```python
from build123d import *

# Parameters (mm, degrees)
SKETCH1_R           = 50
BOSS_EXTRUDE1_DEPTH = 16
SKETCH2_R           = 50
SKETCH2_R_2         = 46.5
BOSS_EXTRUDE2_DEPTH = 1
SKETCH3_R           = 47
CUT_EXTRUDE1_DEPTH  = 10
SKETCH4_R           = 3.15
BOSS_EXTRUDE3_DEPTH = 7


with BuildPart() as part:
    # Sketch1 → Boss-Extrude1 (new body)
    with BuildSketch(Plane(origin=(0, 0, 0), x_dir=(1, 0, 0), z_dir=(0, 1, 0))):
        Circle(SKETCH1_R)
    extrude(amount=BOSS_EXTRUDE1_DEPTH)

    # Sketch2 → Boss-Extrude2 (add)
    with BuildSketch(Plane(origin=(0, 16, 0), x_dir=(1, 0, 0), z_dir=(0, 1, 0))):
        Circle(SKETCH2_R)
        Circle(SKETCH2_R_2, mode=Mode.SUBTRACT)
    extrude(amount=BOSS_EXTRUDE2_DEPTH)

    # Sketch3 → Cut-Extrude1 (cut)
    with BuildSketch(Plane.XZ):
        Circle(SKETCH3_R)
    extrude(amount=-CUT_EXTRUDE1_DEPTH, mode=Mode.SUBTRACT)

    # Sketch4 → Boss-Extrude3 (add)
    with BuildSketch(Plane(origin=(0, 0, 0), x_dir=(1, 0, 0), z_dir=(0, 1, 0))):
        with BuildLine():
            Line((-47.696960071, 15), (-70, 15))
            Line((-70, 15), (-70, -15))
            Line((-70, -15), (-47.696960071, -15))
            ThreePointArc((-47.696960071, -15), (-50, 0), (-47.696960071, 15))
        make_face()
        with Locations((-60, 0)):
            Circle(SKETCH4_R, mode=Mode.SUBTRACT)
        with BuildLine():
            Line((47.696960071, -15), (70, -15))
            Line((70, -15), (70, 15))
            Line((70, 15), (47.696960071, 15))
            ThreePointArc((47.696960071, 15), (50, 0), (47.696960071, -15))
        make_face()
        with Locations((60, 0)):
            Circle(SKETCH4_R, mode=Mode.SUBTRACT)
    extrude(amount=BOSS_EXTRUDE3_DEPTH)


solid = part.part
```
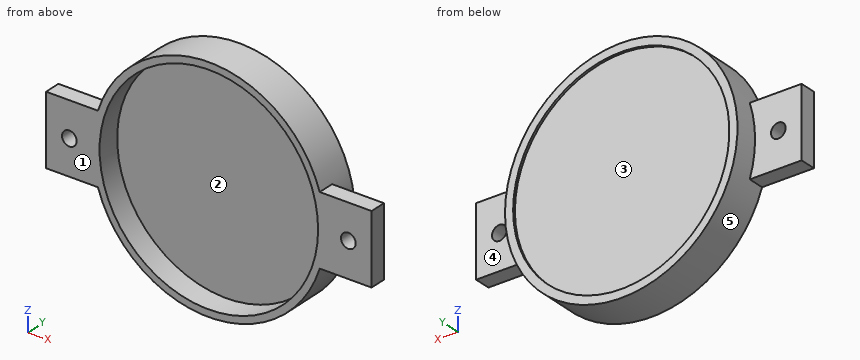
Verification items for the finished model (mm, model axes). Face numbers are marked on the shaded views. A direction names the side the tool comes from. Coordinates: 2 decimals unless noted, no trailing zeros. Loops run counter-clockwise (first coordinate to the right, second up) from the corner with the lowest first, then second, coordinate; pieces in that order, holes last. Notation, with made-up numbers: (-7.75, 48.25) -> (35.25, 48.25) arc R25 cw to (35.25, 82.25) -> close; hole circle Ø7 at (89.25, -4.75). An arc over 180 degrees is marked (long way). Put each result on its own line as item: value.
1. Section check A-A, the plane x = -60. Record the boundary of the cut face in (y, z).
Result set:
outline: (0, -15) -> (7, -15) -> (7, -3.15) -> (0, -3.15) -> close; (0, 3.15) -> (7, 3.15) -> (7, 15) -> (0, 15) -> close
2. Section check B-B, the plane z = 0. Record the boundary of the cut face in (x, y), then the cut area to 3 significant figures.
Result set:
outline: (-70, 0) -> (-63.15, 0) -> (-63.15, 7) -> (-70, 7) -> close; (-56.85, 0) -> (-47, 0) -> (-47, 10) -> (47, 10) -> (47, 0) -> (56.85, 0) -> (56.85, 7) -> (50, 7) -> (50, 17) -> (46.5, 17) -> (46.5, 16) -> (-46.5, 16) -> (-46.5, 17) -> (-50, 17) -> (-50, 7) -> (-56.85, 7) -> close; (63.15, 0) -> (70, 0) -> (70, 7) -> (63.15, 7) -> close
area: 859 mm^2
3. Mould release check, pull along Z, two halves, no side actions. Record for the marked faces 3, 4 and 5: pulls with the +Z half, pulls with the -Z half, needs draft (parallel to the pull), parting line crosses it, or undercut.
Result set:
face 3: undercut
face 4: needs draft
face 5: parting line crosses it
4. Tool access check on the marked faces 1 and 2. Record the directions out of +Z, -Z, +X, -X, +Y, -Y that give a thin tool (end or side, any length) a straight path to the whole face; none if there is none.
Result set:
face 1: +Z, -Z, +X, -X, -Y
face 2: -Y
5. Thickness scan on line 1 (Z direction, x = 0, y = 5.75); line 2 (Z direction, x = 0, y = 16.7); line 3 (Y direction, x = 43.5, z = 12). Record the ranges inside material, lowest first.
Result set:
line 1: z = -50 to -47, 47 to 50
line 2: z = -50 to -46.5, 46.5 to 50
line 3: y = 10 to 16
6. Gauge pin test, flat ends, axial feed: P1, Ø24.5, axis at x = -61, z = 1, coming from the +Y side; P2, Ø2, axis at x = 61.5, y = 4, coming from the -Z side; P3, Ø2, axis at x = 16.5, z = -39, coming from the +Y side; P4, Ø4, axis at x = 32.5, y = 2.5, coming from the -Z side. Record the tip position at first contact, or that the pin passes through.
Result set:
P1: stops at y = 17
P2: stops at z = -15
P3: stops at y = 16
P4: stops at z = -39.62
7. Section check C-C, the plane y = 4.75. Record the boundary of the cut face in (x, z).
Result set:
outline: (-70, -15) -> (-47.7, -15) arc R50 ccw to (47.7, -15) -> (70, -15) -> (70, 15) -> (47.7, 15) arc R50 ccw to (-47.7, 15) -> (-70, 15) -> close; hole circle Ø6.3 at (-60, 0); hole circle Ø94 at (0, 0); hole circle Ø6.3 at (60, 0)
8. Section check D-D, the plane x = -36. Record the boundary of the cut face in (y, z).
Result set:
outline: (0, -34.7) -> (17, -34.7) -> (17, -29.43) -> (16, -29.43) -> (16, 29.43) -> (17, 29.43) -> (17, 34.7) -> (0, 34.7) -> (0, 30.22) -> (10, 30.22) -> (10, -30.22) -> (0, -30.22) -> close
